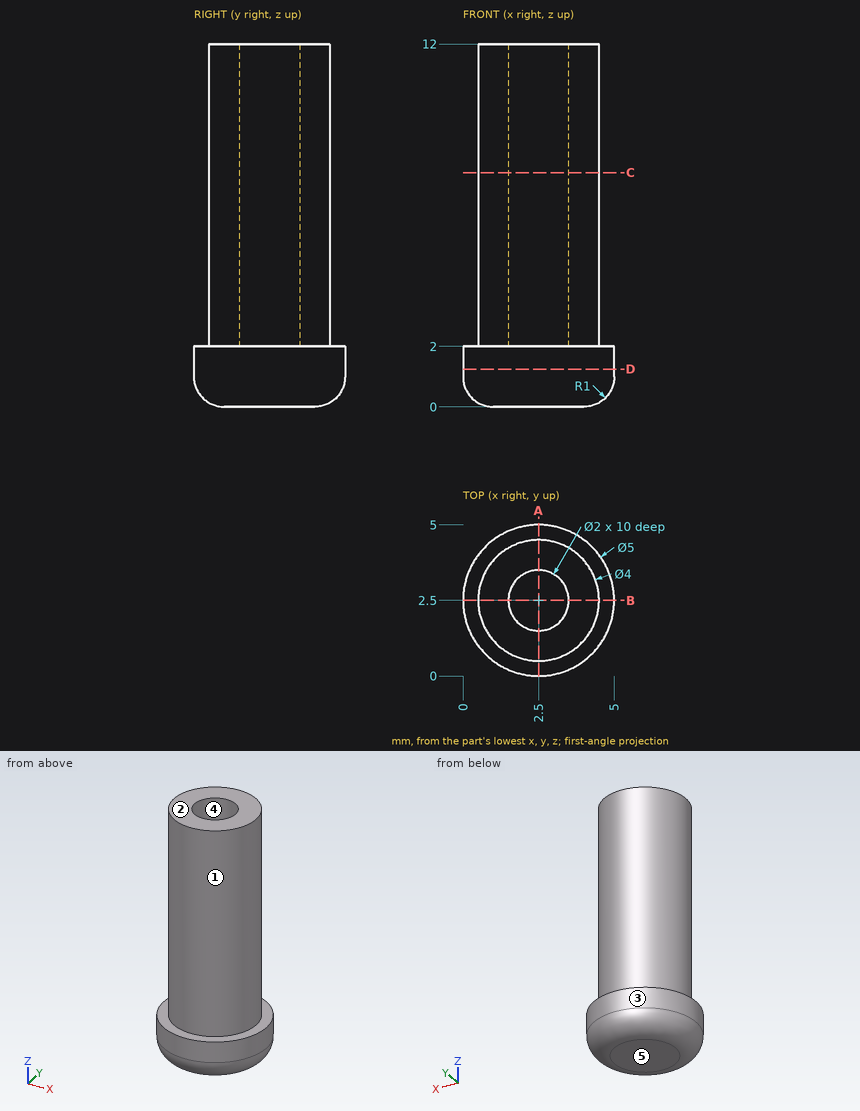
Design review of the part shown in the three views and the two pictorial views. Dimensions are in mm from the part's minimum x, y and z. A direction names the side the tool comes from. Round coordinates to 2 decimals unless told otherwise and drop trailing zeros. Write each loop counter-clockwise with the first axis right and the second up, starting at its lowest first coordinate (ties: lowest second). Pieces come first, ordered by that corner, then holes. Notation, with made-up numbers: (-2, 81) - (8, 81) arc R15 cw to (8, 102) - close; hole circle Ø2 at (51, 87). An arc over 180 degrees is marked (long way). Write item = value, one per line. Start each with the question number.
1. For the marked faces 1 and 2, list the 3-axis set-ups (+Z, -Z, +X, -X, +Y, -Y) from which the entire face can be reached by the end or side of a thin tool; tool diameter is ignored.
2. Wall thickness on L1, parallel to Y at x = 2.5, z = 9; L2, parallel to Z at x = 1.75, y = 1.95; L3, parallel to X at y = 1.65, z = 4: over which ranges is each line inside the solid? List them lowest first.
3. Consider section D-D on z = 1.25. State the section outline as (x, y) points, plus the area to 3 significant figures.
4. Consider section A-A on x = 2.5. State the section outline as (y, z) points.
5. For pin 1 Ø0.6 at (x, y) = (2.5, 2.5) entering from +Z; pin 2 Ø3 at (y, z) = (0.5, 2.5) entering from -X; pin 3 Ø1 at (y, z) = (2, 5.5) entering from +X, all flat-tipped, find the tip position at first contact; note any pin that passes through.
6. Consider section C-C on z = 7.75. State the section outline as (x, y) points, plus the area to 3 significant figures.
7. Draft analysis for pull direction Y (two halves, no side actions). For the marked faces 3, 4 and 5, state which applies: released by +Y, released by -Y, zero draft, split by the parting line, or undercut.
Evaluation:
q1.face_1 = +Z
q1.face_2 = +Z, +X, -X, +Y, -Y
q2.L1 = 0.5 to 1.5, 3.5 to 4.5
q2.L2 = 0 to 2
q2.L3 = 0.69 to 1.97, 3.03 to 4.31
q3.outline = circle Ø5 at (2.5, 2.5)
q3.area = 19.6 mm2
q4.outline = (0, 1) arc R1 ccw to (1, 0) - (4, 0) arc R1 ccw to (5, 1) - (5, 2) - (4.5, 2) - (4.5, 12) - (3.5, 12) - (3.5, 2) - (1.5, 2) - (1.5, 12) - (0.5, 12) - (0.5, 2) - (0, 2) - close
q5.pin_1 = 2
q5.pin_2 = 0.07
q5.pin_3 = 4.5
q6.outline = circle Ø4 at (2.5, 2.5); hole circle Ø2 at (2.5, 2.5)
q6.area = 9.42 mm2
q7.face_3 = split by the parting line
q7.face_4 = undercut
q7.face_5 = zero draft
